The listing builds one solid part. Answer for the finished solid, in the listing's coordinates (mm). A direction names the side the tool comes from. Give positions to 0.01 mm unless a question says otherwise; leave off trailing zeros. Order: outer loops, then holes, each group sorted by start corner. A loop starts at its lowest first (then second) coordinate and runs counter-clockwise, first axis right, second up. Notation, with made-up numbers: M 40.25,42 L 55.25,42 A26 ccw 55.25,74 Z; hole C -19,26.25 d2. An arc over 180 degrees is marked long. Answer as a JSON object with one key per item and string values. Group by question number.
```python
from build123d import *

# Parameters (mm, degrees)
EXTRUDE1_DEPTH     = 53
HOLE1_D            = 13
HOLE1_DEPTH        = 53
SKETCH5_R          = 4
CUT_EXTRUDE1_DEPTH = 4
SKETCH6_R          = 5.5
CUT_EXTRUDE2_DEPTH = 3
SKETCH7_R          = 2
CUT_EXTRUDE3_DEPTH = 33
CUT_EXTRUDE4_DEPTH = 5


with BuildPart() as part:
    # Sketch1 → Extrude1 (new body)
    with BuildSketch(Plane(origin=(0, 0, 0), x_dir=(1, 0, 0), z_dir=(0, 1, 0))):
        with BuildLine():
            Line((-48.427781283, 31), (48.427781283, 31))
            ThreePointArc((48.427781283, 31), (57.5, 0), (48.427781283, -31))
            Line((48.427781283, -31), (-48.427781283, -31))
            ThreePointArc((-48.427781283, -31), (-57.5, 0), (-48.427781283, 31))
        make_face()
    extrude(amount=EXTRUDE1_DEPTH)

    # Sketch2 → Revolve1 (revolve)
    with BuildSketch(Plane.XY, mode=Mode.PRIVATE) as revolve1_sk:
        Polygon((0, 91), (-11.75, 91), (-11.75, 75), (-31, 75), (-31, 53), (0, 53), align=None)
    revolve(revolve1_sk.sketch.rotate(Axis((0, 0, 0), (0, 1, 0)), 270), axis=Axis((0, 0, 0), (0, 1, 0)))  # turned: the seam where the file's is

    # Hole1
    with Locations(Plane(origin=(0, 53, 0), x_dir=(-1, 0, 0), z_dir=(0, 1, 0))):
        with Locations((45, 0), (-45, 0)):
            Hole(HOLE1_D / 2, depth=HOLE1_DEPTH)

    # Sketch5 → Cut-Extrude1 (cut)
    with BuildSketch(Plane.XZ):
        with Locations(Location((0, 0, 0), (0, 0, 270))):  # turned: the seam where the file's is
            Circle(SKETCH5_R)
    extrude(amount=-CUT_EXTRUDE1_DEPTH, mode=Mode.SUBTRACT)

    # Sketch6 → Cut-Extrude2 (cut)
    with BuildSketch(Plane.XZ):
        with Locations(Location((35, -15, 0), (0, 0, 270))):  # turned: the seam where the file's is
            Circle(SKETCH6_R)
    extrude(amount=-CUT_EXTRUDE2_DEPTH, mode=Mode.SUBTRACT)

    # Sketch7 → Cut-Extrude3 (cut)
    with BuildSketch(Plane.XZ.offset(-3)):
        with Locations(Location((35, -15, 0), (0, 0, 270))):  # turned: the seam where the file's is
            Circle(SKETCH7_R)
    extrude(amount=-CUT_EXTRUDE3_DEPTH, mode=Mode.SUBTRACT)

    # Sketch8 → Cut-Revolve1 (revolve, cut)
    with BuildSketch(Plane(origin=(0, 0, 0), x_dir=(0.920504853, 0, -0.390731128), z_dir=(0.390731128, 0, 0.920504853)), mode=Mode.PRIVATE) as cut_revolve1_sk:
        Polygon((57.5, 28), (55, 28), (55, 33.4215), (53.517364509, 34.2775), (35, 34.2775), (35, 40), (57.5, 40), align=None)
    revolve(cut_revolve1_sk.sketch.rotate(Axis((47.484793311, 40, -20.156098913), (-0.920504853, 0, 0.390731128)), 270), axis=Axis((47.484793311, 40, -20.156098913), (-0.920504853, 0, 0.390731128)), mode=Mode.SUBTRACT)  # turned: the seam where the file's is

    # Sketch9 → Revolve2 (revolve)
    with BuildSketch(Plane(origin=(0, 0, 0), x_dir=(0.920504853, 0, -0.390731128), z_dir=(0.390731128, 0, 0.920504853)), mode=Mode.PRIVATE) as revolve2_sk:
        Polygon((55, 31), (55, 34.2775), (46, 34.2775), (45, 35.2775), (45, 40), (60, 40), (60, 31), align=None)
    revolve(revolve2_sk.sketch.rotate(Axis((68.658528533, 40, -29.14381628), (-0.920504853, 0, 0.390731128)), 270), axis=Axis((68.658528533, 40, -29.14381628), (-0.920504853, 0, 0.390731128)))  # turned: the seam where the file's is

    # Sketch10 → Cut-Extrude4 (cut)
    with BuildSketch(Plane(origin=(55.230291207, 0, -23.443867709), x_dir=(-0.390731128, 0, -0.920504853), z_dir=(0.920504853, 0, -0.390731128))):
        Polygon((4.041451884, 40), (2.020725942, 43.5), (-2.020725942, 43.5), (-4.041451884, 40), (-2.020725942, 36.5), (2.020725942, 36.5), align=None)
    extrude(amount=-CUT_EXTRUDE4_DEPTH, mode=Mode.SUBTRACT)


solid = part.part
```
Item 1: Section C-C (y = 17.5) is taken. Determine the outline of the cut face in (x, z).
Item 2: Consider probe 1 along Z at (x, y) = (-45, 32); probe 2 along Z at (x, y) = (35, 31); probe 3 along X at (y, z) = (80.5, -0.5). Determine where each line is inside the solid, lowest interval first. Write a range as from..to.
Item 3: Determine the mould class of faces 6 (the flat face through (-35, 53, 0)), 7 (the cylindrical face through (-30.736, 63.846, 4.036)), 8 (the cylindrical face through (33, 19, -15)) for opening direction Z: released by +Z, released by -Z, zero draft, split by the parting line, or undercut.
Item 4: A tool of negligible diameter and unlimited length cuts with its end or side. For faces 1 (the cylindrical face through (-7.9, 82.9, 8.7)), 2 (the flat face through (32.6, 3, -14.9)), 3 (the flat face through (36, 53, 0)), 4 (the flat face through (51.77, 41.73, -25.28)), 5 (the flat face through (50.65, 40.05, -21.44)), from which of +Z, -Z, +X, -X, +Y, -Y can it reach the whole face along a straight path? Write none if from no direction.
Item 5: Section B-B (z = 0) is taken. Determine the outline of the cut face in (x, y).
Item 6: Section A-A (x = -45) is taken. Determine the outline of the cut face in (y, z), and give its area (3 significant figures).
Item 7: Flat-ended cylindrical pins translate along their axes: P1, Ø2, axis at x = -19.5, y = 72, coming from the +Z side; P2, Ø1.5, axis at x = -25.5, y = 59.5, coming from the +Z side; P3, Ø8, axis at x = 45, z = 0, coming from the -Y side; P4, Ø10, axis at x = 39.5, y = 32.5, coming from the -Z side. Find the tip coordinate at first contact, or state that the pin passes through.
Item 8: Section D-D (x = 2) is taken. Determine the outline of the cut face in (y, z).
Values found:
{
 "1": {"outline": "M -48.43,-31 L 48.43,-31 A57.5 ccw 48.43,31 L -48.43,31 A57.5 ccw Z; hole C -45,0 d13; hole C 35,-15 d4; hole C 45,0 d13"},
 "2": {"probe 1": "z = -31..-6.5, 6.5..31", "probe 2": "z = -31..-17, -13..31", "probe 3": "x = -11.74..11.74"},
 "3": {"face 6": "zero draft", "face 7": "split by the parting line", "face 8": "undercut"},
 "4": {"face 1": "+Y", "face 2": "-Y", "face 3": "+X, +Y", "face 4": "+X", "face 5": "none"},
 "5": {"outline": "M -57.5,0 L -51.5,0 L -51.5,53 L -57.5,53 Z; M -38.5,0 L -4,0 L -4,4 L 4,4 L 4,0 L 38.5,0 L 38.5,53 L 31,53 L 31,75 L 11.75,75 L 11.75,91 L -11.75,91 L -11.75,75 L -31,75 L -31,53 L -38.5,53 Z; M 51.5,0 L 57.5,0 L 57.5,53 L 51.5,53 Z"},
 "6": {"outline": "M 0,-31 L 53,-31 L 53,-6.5 L 0,-6.5 Z; M 0,6.5 L 53,6.5 L 53,31 L 0,31 Z", "area": "2,600 mm^2"},
 "7": {"P1": "stops at z = 24.87", "P2": "stops at z = 18.67", "P3": "passes through", "P4": "stops at z = -31"},
 "8": {"outline": "M 0,-31 L 53,-31 L 53,-30.94 L 75,-30.94 L 75,-11.58 L 91,-11.58 L 91,11.58 L 75,11.58 L 75,30.94 L 53,30.94 L 53,31 L 0,31 L 0,3.46 L 4,3.46 L 4,-3.46 L 0,-3.46 Z"}
}
